Job drawing, mm, ordinate dimensions from the low corner. One solid piece. Give positions to 0.01 mm unless a question says otherwise; leave off trailing zeros. Order: outer loops, then holes, each group sorted by start corner. A loop starts at its lowest first (then second) coordinate and runs counter-clockwise, first axis right, second up.
1. Drop flat-ended pins along their axis: pin 1 Ø1.5 at (x, y) = (24, 3.5) entering from -Z; pin 2 Ø3 at (x, y) = (43.5, 3) entering from +Z; pin 3 Ø6 at (x, y) = (42.5, 8) entering from +Z. Give the stop position or say it passes through.
2. Slice it at C-C on x = 14. List the corners of the cut face in (y, z), and give its area (3 significant figures).
3. Slice it at B-B on x = 50. List the corners of the cut face in (y, z).
4. Probe line 1 (Z direction, x = 33.5, y = 2); line 2 (Z direction, x = 36.5, y = 10.5); line 3 (X direction, y = 8, z = 119.5). List the from-to ranges inside material, lowest first.
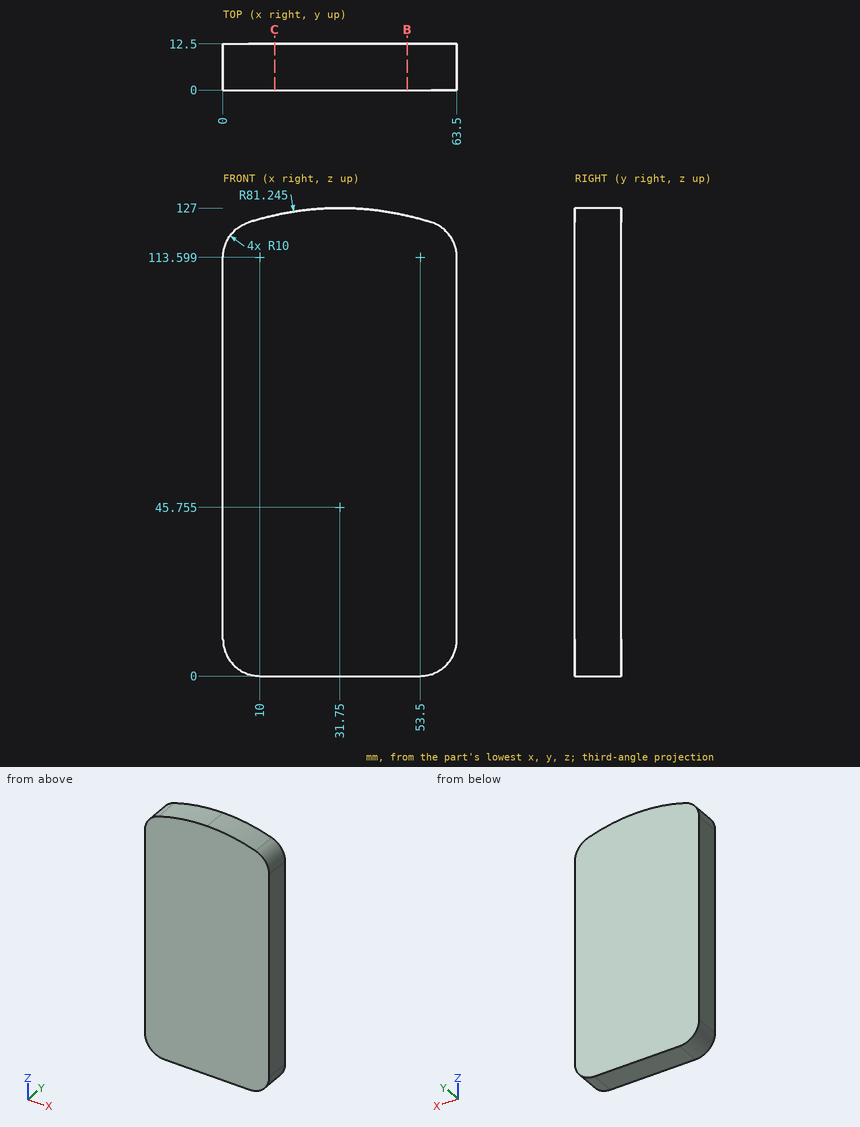
Data:
1. pin 1: stops at z = 0
1. pin 2: stops at z = 126.35
1. pin 3: stops at z = 126.63
2. outline: (0, 0) - (12.5, 0) - (12.5, 125.04) - (0, 125.04) - close
2. area: 1,560 mm2
3. outline: (0, 0) - (12.5, 0) - (12.5, 124.92) - (0, 124.92) - close
4. line 1: z = 0 to 126.98
4. line 2: z = 0 to 126.86
4. line 3: x = 1.93 to 61.57
